Source: CAD feature listing. Evaluate the final solid. Frame: model axes, mm. Round coordinates to 2 decimals unless told otherwise and drop trailing zeros. Loops run counter-clockwise (first coordinate to the right, second up) from the corner with the lowest first, then second, coordinate; pieces in that order, holes last. Notation, with made-up numbers: (88, 17) -> (113, 17) arc R10 cw to (113, 21) -> close; hole circle Ø5 at (14.5, -16.5). An arc over 180 degrees is marked (long way). Write item = value, one per line.
from build123d import *

# Parameters (mm, degrees)
SKETCH1_W           = 230
SKETCH1_H           = 106
SKETCH1_R           = 5
SKETCH1_R_2         = 3.5
SKETCH1_R_3         = 1.75
BOSS_EXTRUDE1_DEPTH = 6


with BuildPart() as part:
    # Sketch1 → Boss-Extrude1 (new body)
    with BuildSketch(Plane(origin=(0, 0, 0), x_dir=(1, 0, 0), z_dir=(0, 1, 0))):
        Rectangle(SKETCH1_W, SKETCH1_H)
        with Locations(Location((0, 0, 0), (0, 0, 270))):
            Circle(SKETCH1_R, mode=Mode.SUBTRACT)
        with Locations(Location((0, 22.25, 0), (0, 0, 270))):
            Circle(SKETCH1_R_2, mode=Mode.SUBTRACT)
        with Locations(Location((0, -22.25, 0), (0, 0, 90))):
            Circle(SKETCH1_R_2, mode=Mode.SUBTRACT)
        with Locations(Location((109, 47, 0), (0, 0, 270))):
            Circle(SKETCH1_R_3, mode=Mode.SUBTRACT)
        with Locations(Location((109, -47, 0), (0, 0, 90))):
            Circle(SKETCH1_R_3, mode=Mode.SUBTRACT)
        with Locations(Location((-109, -47, 0), (0, 0, 270))):
            Circle(SKETCH1_R_3, mode=Mode.SUBTRACT)
        with Locations(Location((-109, 47, 0), (0, 0, 90))):
            Circle(SKETCH1_R_3, mode=Mode.SUBTRACT)
        with Locations(Location((0, 47, 0), (0, 0, 270))):
            Circle(SKETCH1_R_3, mode=Mode.SUBTRACT)
        with Locations(Location((0, -47, 0), (0, 0, 90))):
            Circle(SKETCH1_R_3, mode=Mode.SUBTRACT)
        with BuildLine():
            Line((35, 5), (75, 5))
            ThreePointArc((75, 5), (80, 0), (75, -5))
            Line((75, -5), (35, -5))
            ThreePointArc((35, -5), (30, 0), (35, 5))
        make_face(mode=Mode.SUBTRACT)
        with BuildLine():
            Line((35, 18.75), (75, 18.75))
            ThreePointArc((75, 18.75), (78.5, 22.25), (75, 25.75))
            Line((75, 25.75), (35, 25.75))
            ThreePointArc((35, 25.75), (31.5, 22.25), (35, 18.75))
        make_face(mode=Mode.SUBTRACT)
        with BuildLine():
            Line((16.66, -33.25), (26.66, -33.25))
            ThreePointArc((26.66, -33.25), (28.41, -35), (26.66, -36.75))
            Line((26.66, -36.75), (16.66, -36.75))
            ThreePointArc((16.66, -36.75), (14.91, -35), (16.66, -33.25))
        make_face(mode=Mode.SUBTRACT)
        with BuildLine():
            Line((16.66, 36.75), (26.66, 36.75))
            ThreePointArc((26.66, 36.75), (28.41, 35), (26.66, 33.25))
            Line((26.66, 33.25), (16.66, 33.25))
            ThreePointArc((16.66, 33.25), (14.91, 35), (16.66, 36.75))
        make_face(mode=Mode.SUBTRACT)
        with BuildLine():
            Line((102.66, -33.25), (92.66, -33.25))
            ThreePointArc((92.66, -33.25), (90.91, -35), (92.66, -36.75))
            Line((92.66, -36.75), (102.66, -36.75))
            ThreePointArc((102.66, -36.75), (104.41, -35), (102.66, -33.25))
        make_face(mode=Mode.SUBTRACT)
        with BuildLine():
            Line((102.66, 33.25), (92.66, 33.25))
            ThreePointArc((92.66, 33.25), (90.91, 35), (92.66, 36.75))
            Line((92.66, 36.75), (102.66, 36.75))
            ThreePointArc((102.66, 36.75), (104.41, 35), (102.66, 33.25))
        make_face(mode=Mode.SUBTRACT)
        with BuildLine():
            Line((35, -18.75), (75, -18.75))
            ThreePointArc((75, -18.75), (78.5, -22.25), (75, -25.75))
            Line((75, -25.75), (35, -25.75))
            ThreePointArc((35, -25.75), (31.5, -22.25), (35, -18.75))
        make_face(mode=Mode.SUBTRACT)
        with BuildLine():
            Line((-35, 18.75), (-75, 18.75))
            ThreePointArc((-75, 18.75), (-78.5, 22.25), (-75, 25.75))
            Line((-75, 25.75), (-35, 25.75))
            ThreePointArc((-35, 25.75), (-31.5, 22.25), (-35, 18.75))
        make_face(mode=Mode.SUBTRACT)
        with BuildLine():
            Line((-35, -5), (-75, -5))
            ThreePointArc((-75, -5), (-80, 0), (-75, 5))
            Line((-75, 5), (-35, 5))
            ThreePointArc((-35, 5), (-30, 0), (-35, -5))
        make_face(mode=Mode.SUBTRACT)
        with BuildLine():
            Line((-35, -18.75), (-75, -18.75))
            ThreePointArc((-75, -18.75), (-78.5, -22.25), (-75, -25.75))
            Line((-75, -25.75), (-35, -25.75))
            ThreePointArc((-35, -25.75), (-31.5, -22.25), (-35, -18.75))
        make_face(mode=Mode.SUBTRACT)
    extrude(amount=BOSS_EXTRUDE1_DEPTH)


solid = part.part
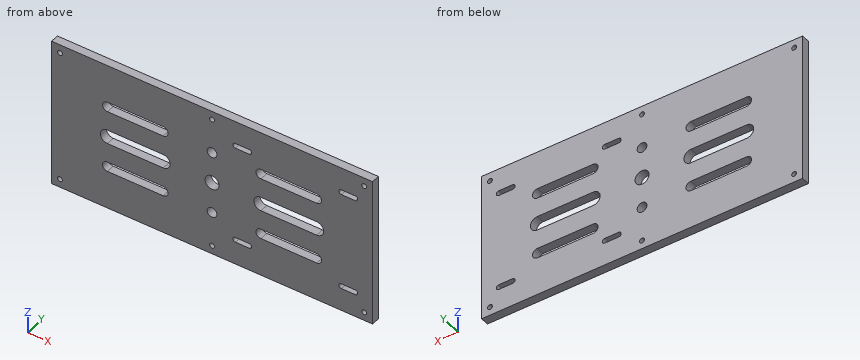
1. Line query: probe 1 along Z at (x, y) = (-47.5, 3.5); probe 2 along Z at (x, y) = (-109, 2.05); probe 3 along Z at (x, y) = (22, 4.8). Output: solid intervals per line, ascending. Write a range as from..to.
Evaluation:
probe_1 = -53..-25.75, -18.75..-5, 5..18.75, 25.75..53
probe_2 = -53..-48.75, -45.25..45.25, 48.75..53
probe_3 = -53..-36.75, -33.25..33.25, 36.75..53
2. Section query B-B (y = 3.55). Give the number of separate pieces and of enclosed holes in the cut face, then the cut area to 3 significant figures.
Evaluation:
separate_pieces = 1
enclosed_holes = 19
area = 21,800 mm²
3. Section query A-A (x = 43). Return the cut outline in (y, z).
Evaluation:
outline = (0, -53) -> (6, -53) -> (6, -25.75) -> (0, -25.75) -> close; (0, -18.75) -> (6, -18.75) -> (6, -5) -> (0, -5) -> close; (0, 5) -> (6, 5) -> (6, 18.75) -> (0, 18.75) -> close; (0, 25.75) -> (6, 25.75) -> (6, 53) -> (0, 53) -> close
